from build123d import *

# Parameters (mm, degrees)
EXTRUDE_THIN1_DEPTH     = 37
CUT_EXTRUDE1_DEPTH      = 119.105884697
CUT_EXTRUDE1_DEPTH_BACK = 119.105884697
CUT_EXTRUDE2_DEPTH      = 119.105884697
BOSS_EXTRUDE1_DEPTH     = 10
SKETCH4_R               = 21
BOSS_EXTRUDE2_DEPTH     = 30
SKETCH5_R               = 17.5
BOSS_EXTRUDE3_DEPTH     = 105
CUT_EXTRUDE3_START      = -64
CUT_EXTRUDE3_DEPTH      = 64


with BuildPart() as part:
    # Sketch1 → Extrude-Thin1 (new, symmetric)
    with BuildSketch(Plane.XY):
        Polygon((-58, -38), (0, -38), (0, 38), (-58, 38), (-58, 48), (10, 48), (10, -48), (-58, -48), align=None)
    extrude(amount=EXTRUDE_THIN1_DEPTH, both=True)

    # Sketch2 → Cut-Extrude1 (cut, two sides: drawn at the far end of the back side and taken through both)
    with BuildSketch(Plane(origin=(0, 48, 0), x_dir=(1, 0, 0), z_dir=(0, 1, 0)).offset(-CUT_EXTRUDE1_DEPTH_BACK)):
        with BuildLine():
            Line((-49.370277543, 13.632170103), (0, 37))
            Line((0, 37), (-58, 37))
            Line((-58, 37), (-58, 5.3e-08))
            ThreePointArc((-58, 5.3e-08), (-55.661233981, 8.06703435), (-49.370277543, 13.632170103))
        make_face()
        with BuildLine():
            ThreePointArc((-49.370277543, -13.632170103), (-55.661234009, -8.067034306), (-58, 5.3e-08))
            Line((-58, 5.3e-08), (-58, -37))
            Line((-58, -37), (0, -37))
            Line((0, -37), (-49.370277543, -13.632170103))
        make_face()
    extrude(amount=CUT_EXTRUDE1_DEPTH + CUT_EXTRUDE1_DEPTH_BACK, mode=Mode.SUBTRACT)

    # Sketch2_3 → Cut-Extrude2 (cut, through all)
    with BuildSketch(Plane(origin=(0, 48, 0), x_dir=(1, 0, 0), z_dir=(0, 1, 0))):
        with BuildLine():
            ThreePointArc((-47.917929128, 0), (-42.917929128, -5), (-37.917929128, 0))
            Line((-37.917929128, 0), (-47.917929128, 0))
        make_face()
        with BuildLine():
            Line((-47.917929128, 0), (-37.917929128, 0))
            ThreePointArc((-37.917929128, 0), (-42.917929128, 5), (-47.917929128, 0))
        make_face()
    extrude(amount=-CUT_EXTRUDE2_DEPTH, mode=Mode.SUBTRACT)

    # Sketch3 → Boss-Extrude1 (add)
    with BuildSketch(Plane(origin=(10, 0, 0), x_dir=(0, 0, -1), z_dir=(1, 0, 0))):
        with BuildLine():
            Line((-14.966629547, 26), (14.966629547, 26))
            ThreePointArc((14.966629547, 26), (30, 0), (14.966629547, -26))
            Line((14.966629547, -26), (-14.966629547, -26))
            ThreePointArc((-14.966629547, -26), (-30, 0), (-14.966629547, 26))
        make_face()
    extrude(amount=BOSS_EXTRUDE1_DEPTH)

    # Sketch4 → Boss-Extrude2 (add)
    with BuildSketch(Plane(origin=(20, 0, 0), x_dir=(0, 0, -1), z_dir=(1, 0, 0))):
        with Locations(Location((0, 0, 0), (0, 0, 90))):
            Circle(SKETCH4_R)
    extrude(amount=BOSS_EXTRUDE2_DEPTH)

    # Sketch5 → Boss-Extrude3 (add)
    with BuildSketch(Plane(origin=(50, 0, 0), x_dir=(0, 0, -1), z_dir=(1, 0, 0))):
        with Locations(Location((0, 0, 0), (0, 0, 90))):
            Circle(SKETCH5_R)
    extrude(amount=BOSS_EXTRUDE3_DEPTH)

    # Sketch6 → Cut-Extrude3 (cut)
    with BuildSketch(Plane(origin=(155, 0, 0), x_dir=(0, 0, -1), z_dir=(1, 0, 0)).offset(CUT_EXTRUDE3_START)):
        with BuildLine():
            Line((-15.811388301, 7.5), (15.811388301, 7.5))
            ThreePointArc((15.811388301, 7.5), (0, 17.5), (-15.811388301, 7.5))
        make_face()
    extrude(amount=CUT_EXTRUDE3_DEPTH, mode=Mode.SUBTRACT)


solid = part.part
Source: CAD feature listing. Evaluate the final solid. Frame: model axes, mm. A direction names the side the tool comes from. Round coordinates to 2 decimals unless told otherwise and drop trailing zeros. Loops run counter-clockwise (first coordinate to the right, second up) from the corner with the lowest first, then second, coordinate; pieces in that order, holes last.
Q1. Section B-B, the plane y = -40.5. Return loops of the section in (x, z), plus the area to 3 significant figures.
Q2. Ray query, line 1 (X direction, y = -45, z = 0); line 2 (Y direction, x = -7.5, z = 1); line 3 (X direction, y = -16, z = -15.5). Return the intervals inside material, ascending.
Q3. Section D-D, the plane z = 24. Return loops of the section in (x, y).
Q4. Access query for faces 4 (the face through (15, -26, 0)), 5 (the face through (10, 33, 1)), 6 (the face through (123, 7.5, 0)), 7 (the face through (15, 0, -30)). Directions: +Z, -Z, +X, -X, +Y, -Y. A direction counts if a zero-diameter tool reaches every point of the face in a straight line with its end or side. Return the directions, or none.
Q5. First-contact query: P1, Ø6, axis at y = -20.5, z = 22.5, coming from the -X side; P2, Ø11, axis at x = 14, z = 0.5, coming from the -Y side; P3, Ø3, axis at y = -17.5, z = 10, coming from the +X side; P4, Ø6, axis at x = -42.92, z = 0, coming from the +Y side. Flat tips, straight axial feed; report the tip coordinate or a pass-through.
Q6. Section C-C, the plane y = 0. Return loops of the section in (x, z), plus the area to 4 significant figures.
Q7. Section A-A, the plane x = -35.5. Return loops of the section in (y, z).
Q8. Mould query, pull axis Z, two halves, no side actions, for faces 1 (the face through (15, 26, 0)), 2 (the face through (-24.3, -43.1, 25.5)), 3 (the face through (-47.913, 43.07, -0.22)). Classes: pulls with the +Z half, pulls with the -Z half, needs draft (parallel to the pull), parting line crosses it, or undercut.
Solutions:
1. outline: (-49.37, -13.63) - (0, -37) - (10, -37) - (10, 37) - (0, 37) - (-49.37, 13.63) arc R15.08 ccw to start; hole circle Ø10 at (-42.92, 0)
1. area: 3,330 mm2
2. line 1: x = -58 to -47.92, -37.92 to 10
2. line 2: y = -48 to -38, 38 to 48
2. line 3: x = 0 to 20
3. outline: (-27.47, -48) - (10, -48) - (10, -18) - (20, -18) - (20, 18) - (10, 18) - (10, 48) - (-27.47, 48) - (-27.47, 38) - (0, 38) - (0, -38) - (-27.47, -38) - close
4. face 4: +Z, -Z, +X, -Y
4. face 5: +X
4. face 6: +Z, -Z, +X, +Y
4. face 7: -Z, +X
5. P1: stops at x = 0
5. P2: stops at y = -48
5. P3: stops at x = 50
5. P4: passes through
6. outline: (0, -37) - (10, -37) - (10, -30) - (20, -30) - (20, -21) - (50, -21) - (50, -17.5) - (155, -17.5) - (155, 17.5) - (50, 17.5) - (50, 21) - (20, 21) - (20, 30) - (10, 30) - (10, 37) - (0, 37) - close
6. area: 6,275 mm2
7. outline: (-48, -20.2) - (-38, -20.2) - (-38, 20.2) - (-48, 20.2) - close; (38, -20.2) - (48, -20.2) - (48, 20.2) - (38, 20.2) - close
8. face 1: needs draft
8. face 2: pulls with the +Z half
8. face 3: undercut
